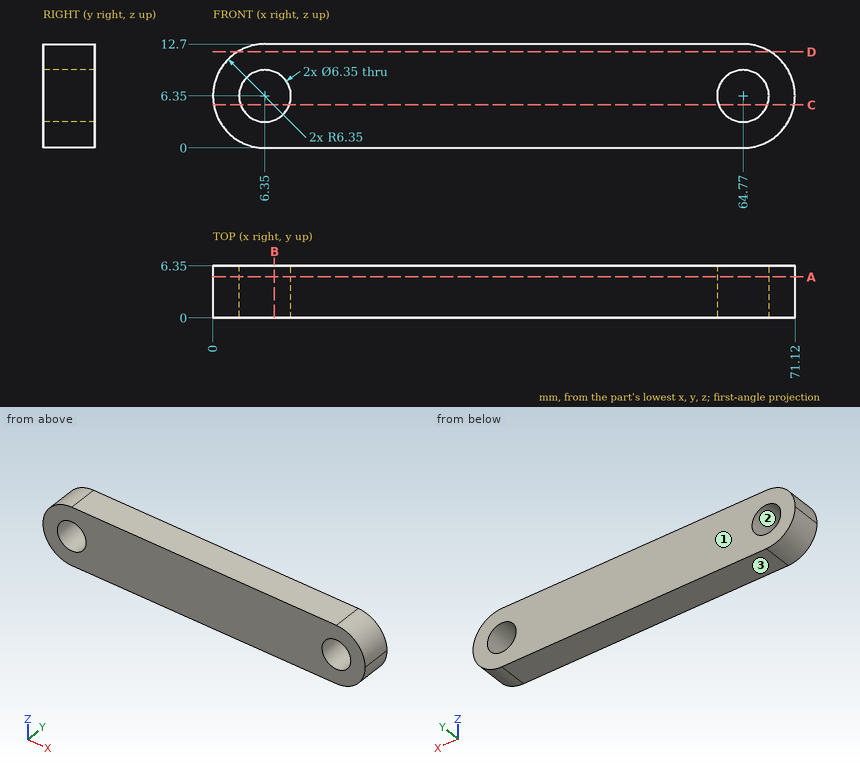
Could you check a few things on this drawing? It's one solid part, dimensions in mm from its lowest x, y, z. Coordinates: 2 decimals unless noted, no trailing zeros. Order: outer loops, then holes, each group sorted by start corner. A loop starts at its lowest first (then second) coordinate and runs counter-clockwise, first axis right, second up.
1. If we section it at C-C (z = 5.25): Please give me the cut outline in (x, y), then the cut area to 3 significant figures.
2. If we section it at A-A (y = 5): Please give me the cut outline in (x, z) (3 decimals).
3. If we section it at D-D (z = 11.75): Please give me the cut outline in (x, y), then the cut area to 3 significant figures.
4. If we section it at B-B (x = 7.5): Please give me the cut outline in (y, z).
5. Thinking about a two-plate mould opening in Z: for the marked faces 1, 2 and 3, which applies, +Z half, -Z half, draft (parallel to the pull), parting line (faces both ways), or undercut?
6. I need wall thicknesses on line 1 (X direction, y = 5.5, z = 3.5); line 2 (X direction, y = 1, z = 5.25); line 3 (Z direction, x = 6, y = 4). Which ranges of each line are inside material? Lowest first, please.
7. I'm going to push flat-ended pins straight in: pin 1 (2 mm diameter, centred on y = 1.5, z = 4.5, fed in from -X); pin 2 (1.5 mm diameter, centred on y = 3, z = 1.5, fed in from -X). Where does each tip first touch, or does it pass through?
Entries:
1. outline: (0.1, 0) - (3.37, 0) - (3.37, 6.35) - (0.1, 6.35) - close; (9.33, 0) - (61.79, 0) - (61.79, 6.35) - (9.33, 6.35) - close; (67.75, 0) - (71.02, 0) - (71.02, 6.35) - (67.75, 6.35) - close
1. area: 375 mm2
2. outline: (6.35, 0) - (64.77, 0) arc R6.35 ccw to (64.77, 12.7) - (6.35, 12.7) arc R6.35 ccw to start; hole circle Ø6.35 at (6.35, 6.35); hole circle Ø6.35 at (64.77, 6.35)
3. outline: (3.01, 0) - (68.11, 0) - (68.11, 6.35) - (3.01, 6.35) - close
3. area: 413 mm2
4. outline: (0, 0) - (6.35, 0) - (6.35, 3.39) - (0, 3.39) - close; (0, 9.31) - (6.35, 9.31) - (6.35, 12.7) - (0, 12.7) - close
5. face 1: draft
5. face 2: undercut
5. face 3: -Z half
6. line 1: x = 0.68 to 4.95, 7.75 to 63.37, 66.17 to 70.44
6. line 2: x = 0.1 to 3.37, 9.33 to 61.79, 67.75 to 71.02
6. line 3: z = 0.01 to 3.19, 9.51 to 12.69
7. pin 1: stops at x = 0.06
7. pin 2: stops at x = 1.5
